Input: dimensioned drawing with shaded views. Units: mm. Origin: part minimum x, y, z. A direction names the side the tool comes from. Give positions to 0.01 mm unless a question says otherwise; leave off trailing zeros. Loops run counter-clockwise (first coordinate to the right, second up) from the corner with the lowest first, then second, coordinate; pieces in that order, holes last.
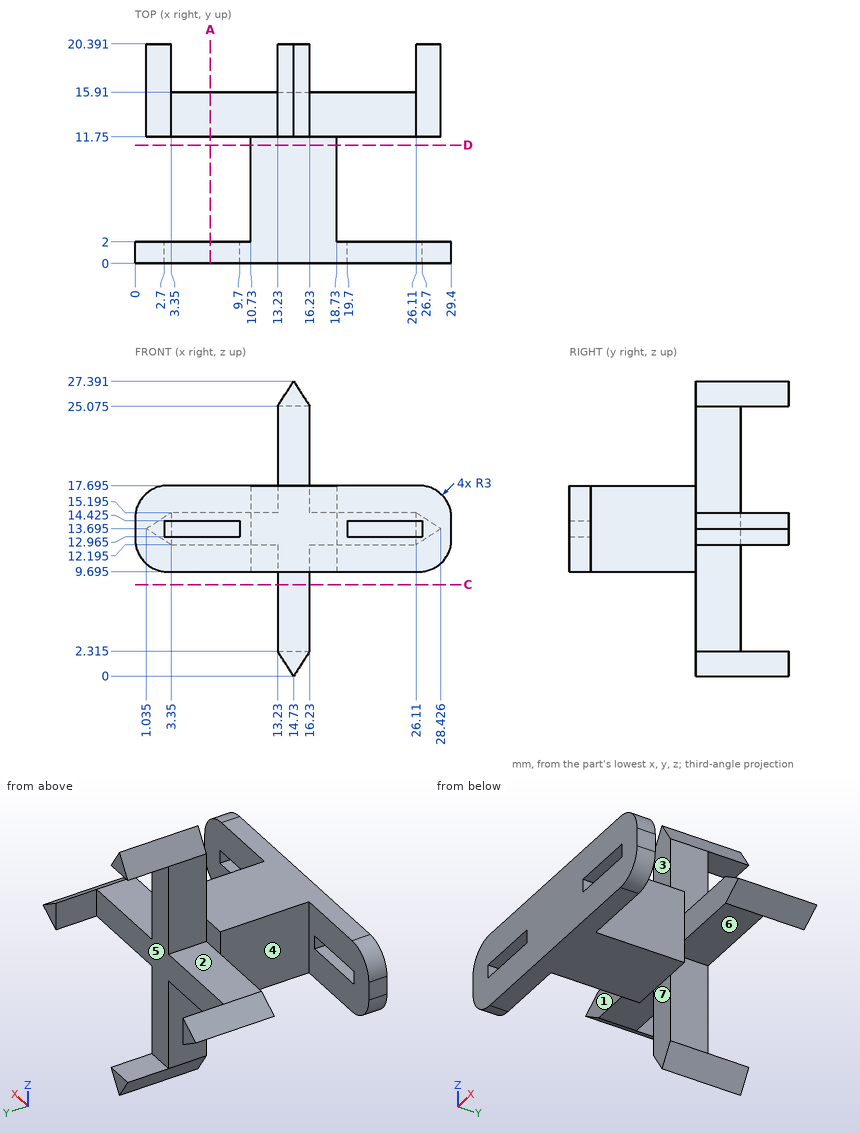
Item 1: Pin query (flat end, axial travel): pin 1 (3 mm diameter, centred on x = 11.5, z = 10.5, fed in from +Y); pin 2 (9 mm diameter, centred on x = 24.5, z = 12.5, fed in from +Y); pin 3 (1.2 mm diameter, centred on x = 19, y = 14, fed in from -Z) (1 decimal); pin 4 (1.5 mm diameter, centred on x = 15, y = 10.5, fed in from -Z) (1 decimal). Return the tip coordinate at first contact, or that it passes through.
Values follow:
pin 1: stops at y = 11.75
pin 2: stops at y = 20.39
pin 3: stops at z = 12.2
pin 4: stops at z = 9.7
Item 2: Section query D-D on y = 11. Return loops of the section in (x, z) (1 decimal), plus the area to 3 significant figures.
Values follow:
outline: (10.7, 9.7) - (18.7, 9.7) - (18.7, 17.7) - (10.7, 17.7) - close
area: 64.0 mm2
Item 3: Set-up query: the marked faces 1, 2 and 3. Return all of +Z, -Z, +X, -X, +Y, -Y with unobstructed straight access to the full face (end or side cutting, diameter ignored); none if empty.
Values follow:
face 1: +Z, -Z, -X
face 2: +Z, -X, +Y
face 3: +Z, +X, -X, -Y
Item 4: Ray query, probe 1 along Z at (x, y) = (23, 1.5) (1 decimal); probe 2 along Y at (x, z) = (9, 12.25); probe 3 along Z at (x, y) = (20.5, 15.5) (1 decimal). Return the intervals inside material, ascending.
Values follow:
probe 1: z = 9.7 to 13, 14.4 to 17.7
probe 2: y = 0 to 2, 11.75 to 15.91
probe 3: z = 12.2 to 15.2
Item 5: Section query A-A on x = 7. Give the number of separate pieces and of enclosed holes in the cut face.
Values follow:
separate pieces: 3
enclosed holes: 0
Item 6: Section query C-C on z = 8.5. Return loops of the section in (x, y), plus the area to 3 significant figures.
Values follow:
outline: (13.23, 11.75) - (16.23, 11.75) - (16.23, 15.91) - (13.23, 15.91) - close
area: 12.5 mm2
Item 7: Draft query along Y for the marked faces 4, 5, 6 and 7. Return one class per face: +Y half, -Y half, draft (parallel to the pull), parting line (faces both ways), or undercut.
Values follow:
face 4: undercut
face 5: +Y half
face 6: draft
face 7: -Y half
